Design review of the part built by this model. Coordinates are the model's own, in mm. Face numbers are marked on the shaded views. A direction names the side the tool comes from. Round coordinates to 2 decimals unless told otherwise and drop trailing zeros. Order: outer loops, then holes, each group sorted by start corner. A loop starts at its lowest first (then second) coordinate and runs counter-clockwise, first axis right, second up. Notation, with made-up numbers: (-6.5, -9.5) - (-2.5, -9.5) arc R23 cw to (-2.5, 18.5) - close; hole circle Ø5 at (-10.75, -34.75). An arc over 180 degrees is marked (long way). Write item = value, one per line.
from build123d import *

# Parameters (mm, degrees)
AUFSATZ_LINEAR_AUSTRAGEN3_DEPTH = 2.8
VERRUNDUNG2_R                   = 0.4
VERRUNDUNG5_R                   = 1.2
VERRUNDUNG6_R                   = 1.2
LINEARES_MUSTER1_COUNT          = 5
LINEARES_MUSTER1_PITCH          = 3.2
SKIZZE5_W                       = 4
SKIZZE5_H                       = 4
AUFSATZ_LINEAR_AUSTRAGEN4_DEPTH = 2.8
VERRUNDUNG3_R                   = 0.4
VERRUNDUNG4_R                   = 0.4
VERRUNDUNG8_R                   = 1.2


# Read off the part's stored shape, not the designer's step: Aufsatz-Linear austragen3
with BuildPart() as part:
    # Aufsatz-Linear austragen3 outline → Aufsatz-Linear austragen3 (new body)
    with BuildSketch(Plane(origin=(84.3, 0, 0), x_dir=(0, 0, -1), z_dir=(1, 0, 0))):
        Polygon((11.9, 5.1), (11.9, 6.3), (11.1, 6.3), (11.1, 4.3), (12.7, 4.3), (12.7, 3.5), (9.5, 3.5), (9.5, 1.1), (12.7, 1.1), (12.7, -0.1), (13.5, -0.1), (13.5, 1.9), (10.3, 1.9), (10.3, 2.7), (13.5, 2.7), (13.5, 5.1), align=None)
    extrude(amount=AUFSATZ_LINEAR_AUSTRAGEN3_DEPTH)

    # Verrundung2
    verrundung2_edges = [part.edges().sort_by_distance(p)[0] for p in [
        (85.7, 1.9, -10.3),
        (85.7, 2.7, -10.3),
        (85.7, 3.5, -12.7),
        (85.7, 4.3, -12.7),
        (85.7, 5.1, -11.9),
        (85.7, 6.3, -11.1),
        (85.7, 6.3, -11.9),
        (85.7, 1.1, -12.7),
    ]]
    fillet(verrundung2_edges, radius=VERRUNDUNG2_R - 0.0001)  # a hair under: the kernel refuses the full size


with BuildPart() as body_2:
    # Abspalten1: the piece on the far side of the plane
    add(part.part)
    split(bisect_by=Plane.ZX.offset(3.5), keep=Keep.BOTTOM)

    # Verrundung5
    verrundung5_edges = [body_2.edges().sort_by_distance(p)[0] for p in [
        (85.7, 1.1, -9.5),
        (85.7, 3.5, -9.5),
    ]]
    fillet(verrundung5_edges, radius=VERRUNDUNG5_R - 0.0001)  # a hair under: the kernel refuses the full size


with BuildPart() as part_1:
    add(part.part)

    # Abspalten1
    split(bisect_by=Plane.ZX.offset(3.5), keep=Keep.TOP)

    # Verrundung6
    verrundung6_edges = [part_1.edges().sort_by_distance(p)[0] for p in [
        (85.7, 5.1, -13.5),
    ]]
    fillet(verrundung6_edges, radius=VERRUNDUNG6_R)


with BuildPart() as lineares_muster1_1:
    # Lineares Muster1: pattern copy
    add(body_2.part.moved(Location(Vector(0, -1, 0) * (1 * LINEARES_MUSTER1_PITCH))))


with BuildPart() as lineares_muster1_2:
    # Lineares Muster1: pattern copy
    add(body_2.part.moved(Location(Vector(0, -1, 0) * (2 * LINEARES_MUSTER1_PITCH))))


with BuildPart() as lineares_muster1_3:
    # Lineares Muster1: pattern copy
    add(body_2.part.moved(Location(Vector(0, -1, 0) * (3 * LINEARES_MUSTER1_PITCH))))


with BuildPart() as lineares_muster1_4:
    # Lineares Muster1: pattern copy
    add(body_2.part.moved(Location(Vector(0, -1, 0) * (4 * LINEARES_MUSTER1_PITCH))))

    # Skizze5 → Aufsatz-Linear austragen4 (add)
    with BuildSketch(Plane(origin=(84.3, 0, 0), x_dir=(0, 0, -1), z_dir=(1, 0, 0))):
        with Locations((11.5, -14.9)):
            Rectangle(SKIZZE5_W, SKIZZE5_H)
        with Locations((11.5, 3.1)):
            Rectangle(SKIZZE5_W, SKIZZE5_H)
    extrude(amount=AUFSATZ_LINEAR_AUSTRAGEN4_DEPTH)


with BuildPart() as aufsatz_linear_austragen4_piece_1:
    # of the separate pieces the step leaves, piece 1, a body of its own (aufsatz_linear_austragen4_pieces)
    add(lineares_muster1_4.part.solids().sort_by_distance((84.3, -9.3, -10.6999))[0])

    # Verrundung3
    verrundung3_edges = [aufsatz_linear_austragen4_piece_1.edges().sort_by_distance(p)[0] for p in [
        (85.7, -12.9, -12.7),
    ]]
    fillet(verrundung3_edges, radius=VERRUNDUNG3_R)


with BuildPart() as aufsatz_linear_austragen4_piece_2:
    # of the separate pieces the step leaves, piece 2, a body of its own (aufsatz_linear_austragen4_pieces)
    add(lineares_muster1_4.part.solids().sort_by_distance((84.3, 1.1, -9.5))[0])


with BuildPart() as part_2:
    add(part_1.part)

    # Kombinieren1: union body 2, Lineares Muster1_1, Lineares Muster1_2, Lineares Muster1_3, Aufsatz-Linear austragen4 piece 1, Aufsatz-Linear austragen4 piece 2
    add(body_2.part)
    add(lineares_muster1_1.part)
    add(lineares_muster1_2.part)
    add(lineares_muster1_3.part)
    add(aufsatz_linear_austragen4_piece_1.part)
    add(aufsatz_linear_austragen4_piece_2.part)

    # Verrundung4
    verrundung4_edges = [part_2.edges().sort_by_distance(p)[0] for p in [
        (85.7, 5.1, -11.1),
        (85.7, 5.1, -13.5),
        (85.7, 0.3, -12.7),
        (85.7, -2.9, -12.7),
        (85.7, -6.1, -12.7),
        (85.7, -9.3, -12.7),
        (85.7, 5.1, -9.5),
    ]]
    fillet(verrundung4_edges, radius=VERRUNDUNG4_R)

    # Verrundung8
    verrundung8_edges = [part_2.edges().sort_by_distance(p)[0] for p in [
        (85.7, -0.5, -13.5),
        (85.7, -3.7, -13.5),
        (85.7, -1.3, -13.5),
        (85.7, -6.9, -13.5),
        (85.7, -4.5, -13.5),
        (85.7, -10.1, -13.5),
        (85.7, -7.7, -13.5),
        (85.7, -10.9, -13.5),
    ]]
    fillet(verrundung8_edges, radius=VERRUNDUNG8_R - 0.0001)  # a hair under: the kernel refuses the full size


solid = part_2.part
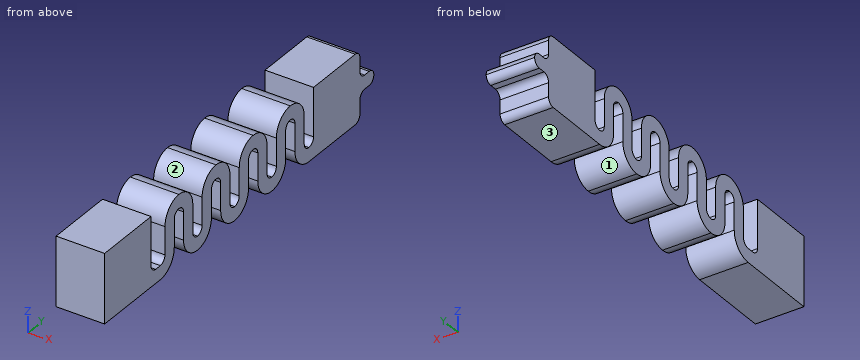
1) We need section B-B on y = -4.75. Write out the cut boundary in (x, z).
Findings:
outline = (84.3, -13.03) - (87.1, -13.03) - (87.1, -9.69) - (84.3, -9.69) - close
2) We need section A-A on z = -12.9. Write out the cut boundary in (x, y), and give its area (3 significant figures).
Findings:
outline = (84.3, -16.9) - (87.1, -16.9) - (87.1, -11.06) - (84.3, -11.06) - close; (84.3, -9.94) - (87.1, -9.94) - (87.1, -7.86) - (84.3, -7.86) - close; (84.3, -6.74) - (87.1, -6.74) - (87.1, -4.66) - (84.3, -4.66) - close; (84.3, -3.54) - (87.1, -3.54) - (87.1, -1.46) - (84.3, -1.46) - close; (84.3, -0.34) - (87.1, -0.34) - (87.1, 5.1) - (84.3, 5.1) - close
area = 49.0 mm^2
3) For the marked faces 1, 2 and 3, list the 3-axis set-ups (+Z, -Z, +X, -X, +Y, -Y) from which the entire face can be reached by the end or side of a thin tool; tool diameter is ignored.
Findings:
face_1 = -Z, +X, -X
face_2 = +Z, +X, -X
face_3 = -Z, +X, -X, +Y, -Y
4) We need section C-C on y = -1.75. Write out the cut boundary in (x, z).
Findings:
outline = (84.3, -13.24) - (87.1, -13.24) - (87.1, -9.85) - (84.3, -9.85) - close
5) To check wall thickness, follow L1, parallel to Y at x = 85.75, z = -13.25; L2, parallel to Y at x = 85.65, z = -9.9; L3, parallel to Y at x = 85.4, z = -13.2. State the ranges of each line that lie inside material, in increasing order. Write a range as from..to.
Findings:
L1 = -16.9..-11.37, -9.63..-8.17, -6.43..-4.97, -3.23..-1.77, -0.03..5.07
L2 = -16.9..-12.9, -11.39..-9.61, -8.19..-6.41, -4.99..-3.21, -1.79..-0.01, 1.1..5.1
L3 = -16.9..-11.31, -9.69..-8.11, -6.49..-4.91, -3.29..-1.71, -0.09..5.09
6) Clearance check with a flat-ended pin moving along its axis: pin 1 Ø0.8 at (x, z) = (86, -11) entering from +Y. State where the tip first meets the part, or that it passes through.
Findings:
pin_1 = 6.29
